Verification items for the finished model (mm, model axes). A direction names the side the tool comes from. Give positions to 0.01 mm unless a question says otherwise; leave off trailing zeros. Loops run counter-clockwise (first coordinate to the right, second up) from the corner with the lowest first, then second, coordinate; pieces in that order, holes last. Notation, with made-up numbers: (16.5, -29.5) - (51.5, -29.5) arc R11 cw to (51.5, -16.5) - close; hole circle Ø1 at (-12, -40). An arc over 180 degrees is marked (long way). One line per item, written item: value. Start each with the question number.
1. Sectioned sample at B-B (x = 14). Record the cut outline in (y, z).
2. Mould release check, pull along X, two halves, no side actions. Record for faces 1 (the flat face through (-23, 45, 19)), 2 (the flat face through (0, -50, 20)), 3 (the flat face through (-30, -1, 20)): pulls with the +X half, pulls with the -X half, needs draft (parallel to the pull), parting line crosses it, or undercut.
3. Access from +Z, -Z, +X, -X, +Y, -Y to the whole of each face (thin tool, end or side, straight path). Record for faces 4 (the flat face through (25, -45, 37)), 5 (the flat face through (0, 1, 0)).
4. Sectioned sample at A-A (z = 23). Record the cut outline in (x, y).
5. Sectioned sample at C-C (y = 21). Record the cut outline in (x, z), plus the area to 3 significant figures.
6. Gauge pin test, flat ends, axial feed: pin 1 (2.5 mm diameter, centred on x = 24.5, y = 45, fed in from +Z); pin 2 (3.5 mm diameter, centred on x = 14, y = 0, fed in from +Z); pin 3 (5 mm diameter, centred on x = -9.5, y = 28.5, fed in from -Z); pin 4 (0.8 mm diameter, centred on x = 14, y = -0.5, fed in from +Z). Record the tip position at first contact, or that the pin passes through.
7. Sectioned sample at D-D (y = -41). Record the cut outline in (x, z), plus the area to 3 significant figures.
8. Scan lines: L1, parallel to Y at x = 14, z = 5; L2, parallel to Y at x = -19, z = 26; L3, parallel to Y at x = -24.5, z = 26.5. Record each from-to range of solid material in increasing order. Write a range as [from, to].
from build123d import *

# Parameters (mm, degrees)
F0_W      = 60
F0_H      = 100
F1_DEPTH  = 40
F2_T      = -2
F3_W      = 22
F3_H      = 75
F4_DEPTH  = 6
F5_R      = 1.35
F6_DEPTH  = 6
F7_W      = 20
F7_H      = 37
F8_DEPTH  = 6
F9_W      = 20
F9_H      = 2
F10_DEPTH = 25
F11_W     = 15
F11_H     = 34
F12_DEPTH = 6
F13_R     = 1.375
F14_DEPTH = 6
F15_W     = 5
F15_H     = 5
F16_DEPTH = 35


with BuildPart() as f1:
    # F0 (on Top) → F1 (new body)
    with BuildSketch(Plane.XY):
        Rectangle(F0_W, F0_H)
    extrude(amount=F1_DEPTH)

    # F2
    f2_openings = [f1.faces().sort_by_distance(p)[0] for p in [
        (0, 0, 40),
    ]]
    offset(amount=F2_T, openings=f2_openings)

    # F3 (on face) → F4 (join)
    with BuildSketch(Plane.XY.offset(2)):
        with Locations((14, 0)):
            Rectangle(F3_W, F3_H)
    extrude(amount=F4_DEPTH)

    # F5 (on face) → F6 (cut)
    with BuildSketch(Plane.XY.offset(8)):
        with Locations((14, 0)):
            Circle(F5_R)
    extrude(amount=-F6_DEPTH, mode=Mode.SUBTRACT)

    # F7 (on face) → F8 (join)
    with BuildSketch(Plane.XY.offset(2)):
        with Locations((-15.1, -29.5)):
            Rectangle(F7_W, F7_H)
    extrude(amount=F8_DEPTH)

    # F9 (on face) → F10 (join)
    with BuildSketch(Plane.XY.offset(8)):
        with Locations((-15.1, -12)):
            Rectangle(F9_W, F9_H)
    extrude(amount=F10_DEPTH)

    # F11 (on face) → F12 (join)
    with BuildSketch(Plane.XY.offset(2)):
        with Locations((-13.210342, 17)):
            Rectangle(F11_W, F11_H)
    extrude(amount=F12_DEPTH)

    # F13 (on face) → F14 (cut)
    with BuildSketch(Plane.XY.offset(8)):
        with Locations((-13.210342, 27)):
            Circle(F13_R)
    extrude(amount=-F14_DEPTH, mode=Mode.SUBTRACT)

    # F15 (on face) → F16 (join)
    with BuildSketch(Plane.XY.offset(2)):
        with Locations((-25.5, 45.5)):
            Rectangle(F15_W, F15_H)
        with Locations((25.5, 45.5)):
            Rectangle(F15_W, F15_H)
        with Locations((25.5, -45.5)):
            Rectangle(F15_W, F15_H)
    extrude(amount=F16_DEPTH)


solid = f1.part
Results are:
1. outline: (-50, 0) - (50, 0) - (50, 40) - (48, 40) - (48, 2) - (37.5, 2) - (37.5, 8) - (1.35, 8) - (1.35, 2) - (-1.35, 2) - (-1.35, 8) - (-37.5, 8) - (-37.5, 2) - (-48, 2) - (-48, 40) - (-50, 40) - close
2. face 1: undercut
2. face 2: needs draft
2. face 3: pulls with the -X half
3. face 4: +Z
3. face 5: -Z, +X, -X, +Y, -Y
4. outline: (-30, -50) - (30, -50) - (30, 50) - (-30, 50) - close; (-25.1, -13) - (-5.1, -13) - (-5.1, -11) - (-25.1, -11) - close; hole (-28, -48) - (23, -48) - (23, -43) - (28, -43) - (28, 43) - (23, 43) - (23, 48) - (-23, 48) - (-23, 43) - (-28, 43) - close
5. outline: (-30, 0) - (30, 0) - (30, 40) - (28, 40) - (28, 2) - (25, 2) - (25, 8) - (3, 8) - (3, 2) - (-5.71, 2) - (-5.71, 8) - (-20.71, 8) - (-20.71, 2) - (-28, 2) - (-28, 40) - (-30, 40) - close
5. area: 494 mm^2
6. pin 1: stops at z = 37
6. pin 2: stops at z = 8
6. pin 3: stops at z = 0
6. pin 4: stops at z = 2
7. outline: (-30, 0) - (30, 0) - (30, 40) - (28, 40) - (28, 2) - (-5.1, 2) - (-5.1, 8) - (-25.1, 8) - (-25.1, 2) - (-28, 2) - (-28, 40) - (-30, 40) - close
7. area: 392 mm^2
8. L1: y = [-50, -48], [-37.5, -1.35], [1.35, 37.5], [48, 50]
8. L2: y = [-50, -48], [-13, -11], [48, 50]
8. L3: y = [-50, -48], [-13, -11], [43, 50]
